Input: part model. Units: mm. Frame: model coordinates. Face numbers are marked on the shaded views. A direction names the side the tool comes from. Round coordinates to 2 decimals unless told otherwise and drop trailing zeros. Write each loop counter-clockwise with the first axis right and the second up, starting at its lowest first coordinate (ties: lowest second). Pieces come first, ordered by that corner, then holes. Notation, with made-up numbers: (50.5, -8) - (60.5, -8) arc R14 ccw to (60.5, 4) - close; hole circle Ø4 at (-39, 4). An arc over 180 degrees is marked (long way). Use one line per item in the form item = value.
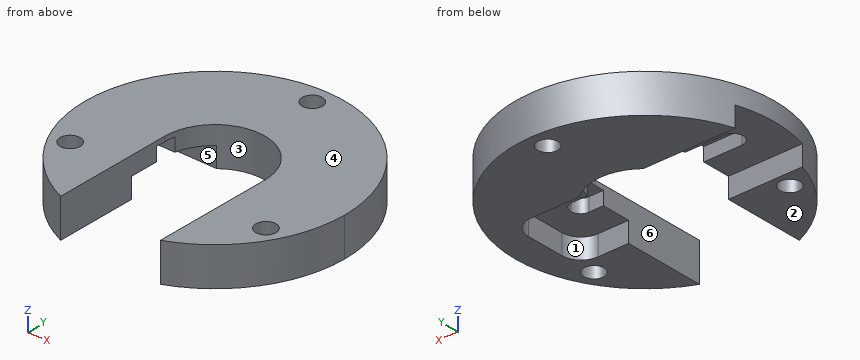
```python
from build123d import *

# Parameters (mm, degrees)
F0_R     = 5.25
F1_DEPTH = 20
F3_DEPTH = 10.5
F4_R     = 10
F6_DEPTH = 7
F8_DEPTH = 7


with BuildPart() as f1:
    # F0 (on Top) → F1 (new body)
    with BuildSketch(Plane.XY):
        with BuildLine():
            ThreePointArc((26, -62.2916527313), (56.1749499332, -37.4249248496), (67.5, 0))
            ThreePointArc((67.5, 0), (-37.4249248496, 56.1749499332), (-26, -62.2916527313))
            Line((-26, -62.2916527313), (-26, 0))
            ThreePointArc((-26, 0), (0, 26), (26, 0))
            Line((26, 0), (26, -62.2916527313))
        make_face()
        with Locations((-51, -28)):
            Circle(F0_R, mode=Mode.SUBTRACT)
        with Locations((51, -28)):
            Circle(F0_R, mode=Mode.SUBTRACT)
        with Locations((0, 58)):
            Circle(F0_R, mode=Mode.SUBTRACT)
    extrude(amount=F1_DEPTH)

    # F2 (on face) → F3 (cut)
    with BuildSketch(Plane(origin=(0, 0, 0), x_dir=(1, 0, 0), z_dir=(0, 0, -1))):
        with BuildLine():
            Line((16.6132477258, -20), (52.0419568735, -20))
            Line((52.0419568735, -20), (52.0419568735, 20))
            Line((52.0419568735, 20), (26, 20))
            Line((26, 20), (26, 0))
            ThreePointArc((26, 0), (23.5366144642, -11.0466184674), (16.6132477258, -20))
        make_face()
        with BuildLine():
            Line((-64.4689847911, -20), (-16.6132477258, -20))
            ThreePointArc((-16.6132477258, -20), (-23.5366144642, -11.0466184674), (-26, 0))
            Line((-26, 0), (-26, 20))
            Line((-26, 20), (-64.4689847911, 20))
            ThreePointArc((-64.4689847911, 20), (-67.5, 0), (-64.4689847911, -20))
        make_face()
    extrude(amount=-F3_DEPTH, mode=Mode.SUBTRACT)

    # F4
    f4_edges = [f1.edges().sort_by_distance(p)[0] for p in [
        (52.041957, 20, 5.25),
        (52.041957, -20, 5.25),
    ]]
    fillet(f4_edges, radius=F4_R)

    # F5 (on face) → F6 (cut)
    with BuildSketch(Plane(origin=(0, 0, 10.5), x_dir=(1, 0, 0), z_dir=(0, 0, -1))):
        with BuildLine():
            ThreePointArc((33.629886806, -5), (37.1654207119, -3.5355339059), (38.629886806, 0))
            ThreePointArc((38.629886806, 0), (37.1654207119, 3.5355339059), (33.629886806, 5))
            ThreePointArc((33.629886806, 5), (28.629886806, 0), (33.629886806, -5))
        make_face()
        with BuildLine():
            ThreePointArc((33.629886806, -5), (28.629886806, 0), (33.629886806, 5))
            Line((33.629886806, 5), (26, 5))
            Line((26, 5), (26, 0))
            ThreePointArc((26, 0), (25.8783910121, -2.511748121), (25.5147016443, -5))
            Line((25.5147016443, -5), (33.629886806, -5))
        make_face()
    extrude(amount=-F6_DEPTH, mode=Mode.SUBTRACT)

    # F7 (on face) → F8 (cut)
    with BuildSketch(Plane(origin=(0, 0, 10.5), x_dir=(1, 0, 0), z_dir=(0, 0, -1))):
        with BuildLine():
            ThreePointArc((-45.8243116736, -5.25), (-42.1120010724, -3.7123106012), (-40.5743116736, 0))
            ThreePointArc((-40.5743116736, 0), (-42.1120010724, 3.7123106012), (-45.8243116736, 5.25))
            ThreePointArc((-45.8243116736, 5.25), (-51.0743116736, 0), (-45.8243116736, -5.25))
        make_face()
        with BuildLine():
            ThreePointArc((-45.8243116736, 5.25), (-42.1120010724, 3.7123106012), (-40.5743116736, 0))
            ThreePointArc((-40.5743116736, 0), (-42.1120010724, -3.7123106012), (-45.8243116736, -5.25))
            Line((-45.8243116736, -5.25), (-25.4644359843, -5.25))
            ThreePointArc((-25.4644359843, -5.25), (-25.8657624631, -2.6386231644), (-26, 0))
            Line((-26, 0), (-26, 5.25))
            Line((-26, 5.25), (-45.8243116736, 5.25))
        make_face()
    extrude(amount=-F8_DEPTH, mode=Mode.SUBTRACT)


solid = f1.part
```
(1) Cut plane D-D on y = 23.5. Output: boundary loops of the cut face in (x, z).
Derived:
outline = (-63.28, 0) - (-11.12, 0) - (-11.12, 20) - (-63.28, 20) - close; (11.12, 0) - (63.28, 0) - (63.28, 20) - (11.12, 20) - close
(2) Draft query along X for the marked faces 1, 2 and 3. Return one class per face: released by +X, released by -X, zero draft, split by the parting line, or undercut.
Derived:
face_1 = released by -X
face_2 = zero draft
face_3 = undercut
(3) Cut plane B-B on x = 0. Output: boundary loops of the cut face in (y, z).
Derived:
outline = (26, 0) - (52.75, 0) - (52.75, 20) - (26, 20) - close; (63.25, 0) - (67.5, 0) - (67.5, 20) - (63.25, 20) - close
(4) First-contact query: pin 1 Ø5 at (x, z) = (-42, 8) entering from +Y; pin 2 Ø6.5 at (x, y) = (-51, -28) entering from +Z; pin 3 Ø5 at (y, z) = (20, 3) entering from +X; pin 4 Ø7.5 at (x, z) = (-38, 12.5) entering from -Y. Flat tips, straight axial feed; report the tip coordinate or a pass-through.
Derived:
pin_1 = 54.74
pin_2 = through
pin_3 = 65.19
pin_4 = -58.17
(5) Material intervals for L1, parallel to Y at x = 0, z = 16.25; L2, parallel to Y at x = 55.5, z = 17.5; L3, parallel to Y at x = 51, z = 5.25, sorted ascending.
Derived:
L1 = 26 to 52.75, 63.25 to 67.5
L2 = -38.42 to -30.7, -25.3 to 38.42
L3 = -44.22 to -33.25, -22.75 to -14.44, 14.44 to 44.22
(6) Cut plane C-C on z = 15.5. Output: boundary loops of the cut face in (x, y).
Derived:
outline = (-45.82, -5.25) arc R5.25 cw to (-45.82, 5.25) - (-25.46, 5.25) arc R26 cw to (25.51, 5) - (33.63, 5) arc R5 cw to (33.63, -5) - (26, -5) - (26, -62.29) arc R67.5 ccw (long way) to (-26, -62.29) - (-26, -5.25) - close; hole circle Ø10.5 at (-51, -28); hole circle Ø10.5 at (0, 58); hole circle Ø10.5 at (51, -28)
(7) Cut plane A-A on z = 6.5. Output: boundary loops of the cut face in (x, y), then the cut area to 3 significant figures.
Derived:
outline = (-64.47, -20) arc R67.5 ccw to (-26, -62.29) - (-26, -20) - close; (-64.47, 20) - (-16.61, 20) arc R26 cw to (16.61, 20) - (42.04, 20) arc R10 cw to (52.04, 10) - (52.04, -10) arc R10 cw to (42.04, -20) - (26, -20) - (26, -62.29) arc R67.5 ccw (long way) to start; hole circle Ø10.5 at (-51, -28); hole circle Ø10.5 at (0, 58); hole circle Ø10.5 at (51, -28)
area = 6,840 mm^2
(8) Access query for the marked faces 4, 5 and 6. Directions: +Z, -Z, +X, -X, +Y, -Y. A direction counts if a zero-diameter tool reaches every point of the face in a straight line with its end or side. Return the directions, or none.
Derived:
face_4 = +Z, +X, -X, +Y, -Y
face_5 = -Z, -X
face_6 = +Z, -Z, -Y
